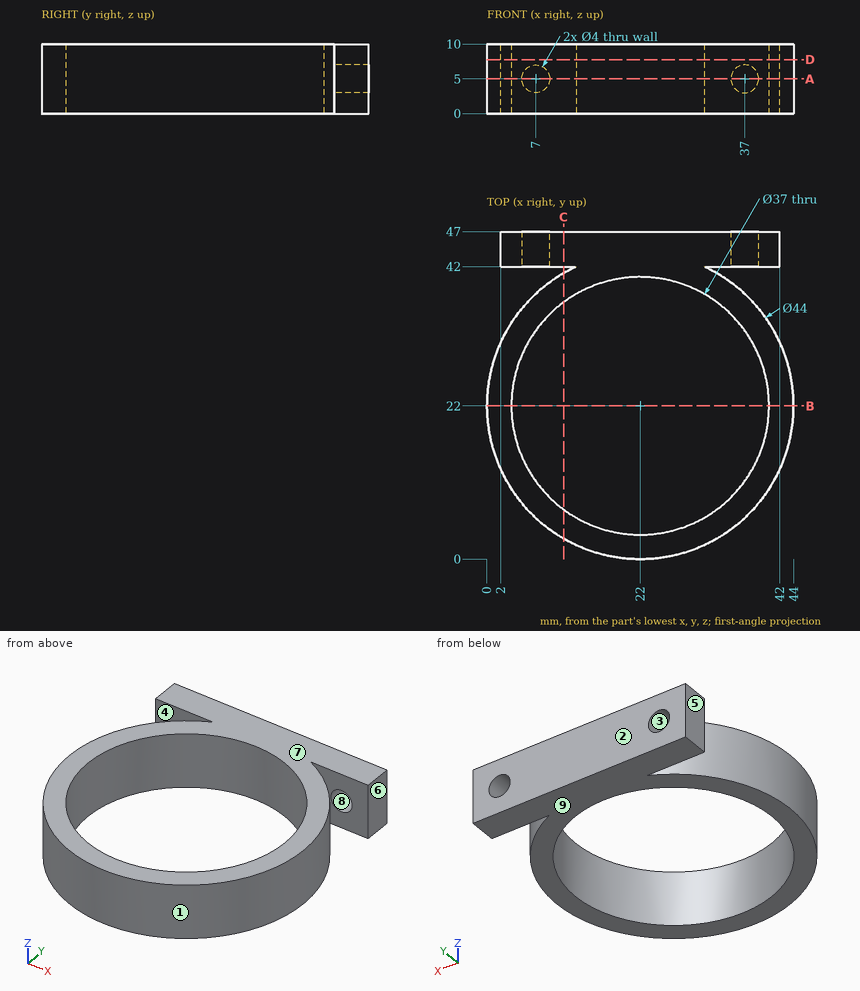
Job drawing, mm, ordinate dimensions from the low corner. One solid piece. A direction names the side the tool comes from. Coordinates: 2 decimals unless noted, no trailing zeros. Order: outer loops, then holes, each group sorted by start corner. A loop starts at its lowest first (then second) coordinate and runs counter-clockwise, first axis right, second up. Notation, with made-up numbers: M 36,42 L 79,42 A33 cw 79,80 Z; hole C -4,71 d5. An arc over 180 degrees is marked long. Return JSON: item names as keys, results as strings.
1. Saw through at D-D (z = 7.75). Give the cut face in (x, y).
Ans:
{"outline": "M 2,42 L 12.83,42 A22 ccw long 31.17,42 L 42,42 L 42,47 L 2,47 Z; hole C 22,22 d37"}
2. Drill centre lines: probe 1 along X at (y, z) = (45.65, 5); probe 2 along Z at (x, y) = (7, 45.9); probe 3 along Y at (x, z) = (22, 3.5). Where is each one in solid material? Low to high.
Ans:
{"probe 1": "2 to 5, 9 to 35, 39 to 42", "probe 2": "0 to 3, 7 to 10", "probe 3": "0 to 3.5, 40.5 to 47"}
3. Flat gauge pins, fed straight in: pin 1 (4 mm diameter, centred on y = 33, z = 3, fed in from +X); pin 2 (3 mm diameter, centred on x = 39, z = 4.5, fed in from -Y); pin 3 (3 mm diameter, centred on y = 12, z = 3, fed in from -X). Where does each tip first touch, or does it go through?
Ans:
{"pin 1": "x = 42.07", "pin 2": "y = 6.39", "pin 3": "x = 1.71"}
4. Saw through at B-B (y = 22). Give the cut face in (x, z), and give its area (3 significant figures).
Ans:
{"outline": "M 0,0 L 3.5,0 L 3.5,10 L 0,10 Z; M 40.5,0 L 44,0 L 44,10 L 40.5,10 Z", "area": "70.0 mm^2"}
5. Saw through at C-C (x = 11). Give the cut face in (y, z).
Ans:
{"outline": "M 2.95,0 L 7.13,0 L 7.13,10 L 2.95,10 Z; M 36.87,0 L 41.05,0 L 41.05,10 L 36.87,10 Z; M 42,0 L 47,0 L 47,10 L 42,10 Z"}
6. Saw through at A-A (z = 5). Give the cut face in (x, y), and give its area (3 significant figures).
Ans:
{"outline": "M 2,42 L 5,42 L 5,47 L 2,47 Z; M 9,42 L 12.83,42 A22 ccw long 31.17,42 L 35,42 L 35,47 L 9,47 Z; M 39,42 L 42,42 L 42,47 L 39,47 Z; hole C 22,22 d37", "area": "581 mm^2"}
7. Pull direction Y, two halves, no side cores. Call the marked faces 1, 2, 3 and 4: +Y half, -Y half, draft (parallel to the pull), parting line (faces both ways), or undercut.
Ans:
{"face 1": "undercut", "face 2": "+Y half", "face 3": "draft", "face 4": "undercut"}
8. Tool access for the marked faces 5, 6, 7, 8 and 9: list every direction of +Z, -Z, +X, -X, +Y, -Y with a clear straight run to the whole face (end or side of a thin tool).
Ans:
{"face 5": "+Z, -Z, -X, +Y", "face 6": "+Z, -Z, +X, +Y", "face 7": "+Z, +X, -X, +Y, -Y", "face 8": "+Y", "face 9": "-Z, +X, -X, +Y, -Y"}
